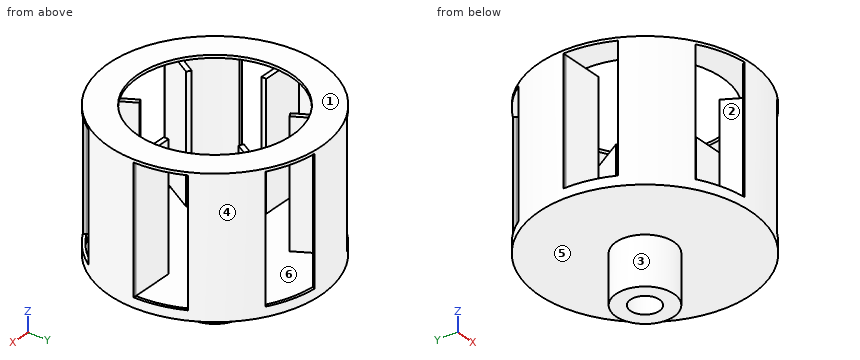
Autodesk Inventor part; units mm, degrees
ref_plane "Work Plane1" through (-58.9042, -102.025, 1.5) normal (-0.5, -0.866, 0) x (0.866, -0.5, 0)
ref_plane "YZ Plane" through (0, 0, 0) normal (1, 0, 0) x (0, 1, 0)
ref_plane "XZ Plane" through (0, 0, 0) normal (0, 1, 0) x (-1, 0, 0)
sketch "Sketch1" plane through (0, 0, 0) normal (0, 0, 1) x (1, 0, 0)
  circle A0 centre (0, 0) radius 55
  dimension "d0" = 110
extrude "Extrusion1" add sketch "Sketch1" along normal blind 71.5
shell "Shell1" thickness 1.5 removed faces 1 at (13.749, -10.4033, 71.5)
sketch "Sketch2" plane through (0, 0, 71.5) normal (0, 0, 1) x (1, 0, 0)
  circle A0 centre (0, 0) radius 55
  circle A1 centre (0, 0) radius 55
  circle A2 centre (0, 0) radius 40
  dimension "d4" = 110
  dimension "d5" = 80
extrude "Extrusion2" add sketch "Sketch2" against normal blind 1.5
sketch "Sketch3" plane through (0, 0, 0) normal (0, 0, -1) x (-1, 0, 0)
  circle A0 centre (0, 0) radius 15
  dimension "d8" = 30
extrude "Extrusion3" add sketch "Sketch3" along normal blind 25
sketch "Sketch4" plane through (0, 0, -25) normal (0, 0, -1) x (-1, 0, 0)
  circle A0 centre (0, 0) radius 7.5
  dimension "d11" = 15
extrude "Extrusion4" cut sketch "Sketch4" against normal blind 25
sketch "Sketch5" plane through (0, 0, 1.5) normal (0, 0, 1) x (1, 0, 0)
  circle A0 centre (0, 0) radius 7.5 construction
  line L0 (0, 0) -> (0, -95.8386) construction
  line L1 (0, 0) -> (-58.9042, -102.025)
  dimension "d14" = 30
ref_plane "Work Plane1" through (-58.9042, -102.025, 1.5) normal (-0.5, -0.866, 0) x (0.866, -0.5, 0)
sketch "Sketch7" plane through (-58.9042, -102.025, 1.5) normal (-0.5, -0.866, 0) x (0.866, -0.5, 0)
  line L0 (53.5, 0) -> (-53.5, 0)
  line L1 (55, -1.5) -> (-55, -1.5)
  line L2 (0, 3.5) -> (24, 3.5)
  line L3 (24, 3.5) -> (24, 68.5)
  line L4 (24, 68.5) -> (0, 68.5)
  line L5 (0, 68.5) -> (0, 3.5)
  line L6 (55, 70) -> (-55, 70)
  point P0 (0, -1.5)
  point P1 (0, -1.5)
  dimension "d18" = 5
  dimension "d19" = 65
  dimension "d20" = 24
  dimension "d21" = 0
  dimension "d22" = 1.5
extrude "Extrusion5" cut sketch "Sketch7" against normal blind 110.75
pattern_circular "Circular Pattern1" count 6 over 360 about axis through (0, 0, 0) along (0, 0, 1) of "Extrusion5"
sketch "Sketch12" plane through (0, 0, 5) normal (0, 0, 1) x (0.958, -0.2869, 0)
  line L0 (9.6549, 29.9119) -> (14.7648, 51.483)
  line L1 (14.7648, 51.483) -> (14.9013, 52.0593)
  line L2 (7.2222, 30.4881) -> (12.3321, 52.0593)
  line L3 (12.3321, 52.0593) -> (12.4686, 52.6356)
  line L4 (14.9013, 52.0593) -> (12.4686, 52.6356)
  line L5 (12.6779, 53.5189) -> (12.3321, 52.0593)
  line L6 (9.6549, 29.9119) -> (7.2222, 30.4881)
  point P0 (0, 0)
  point P1 (8.4385, 30.2)
  dimension "d34" = 2.5
  dimension "d35" = 30.2
extrude "Extrusion7" add sketch "Sketch12" along normal blind 65
pattern_circular "Circular Pattern2" count 6 over 360 about axis through (0, 0, -25) along (0, 0, 1) of "Extrusion7"
properties part number "Cilindro do Motor Industrial" material "Iron, Cast"
Verification items for the finished model (mm, model axes). Face numbers are marked on the shaded views. A direction names the side the tool comes from. Round coordinates to 2 decimals unless told otherwise and drop trailing zeros. Order: outer loops, then holes, each group sorted by start corner. A loop starts at its lowest first (then second) coordinate and runs counter-clockwise, first axis right, second up. Notation, with made-up numbers: (18, -28) - (50, -28) arc R13 cw to (50, -16) - close; hole circle Ø8 at (-27.75, 23.25). An arc over 180 degrees is marked (long way). Use CSV: the item, a comma, the result in double quotes. Start each with the question number.
1) Thickness scan on L1, parallel to Z at x = 21, y = -42.5; L2, parallel to Y at x = 0, z = 34.5; L3, parallel to Y at x = -19.5, z = 14. Record the ranges inside material, lowest first.
2) Section check C-C, the plane z = 58. State how many separate pieces and enclosed holes the cut face has, plus the area to 3 significant figures.
3) Section check D-D, the plane x = 0. Record the cut outline in (y, z), plus the area to 4 significant figures.
4) Section check B-B, the plane x = -35. Record the cut outline in (y, z), plus the area to 3 significant figures.
5) Access from +Z, -Z, +X, -X, +Y, -Y to the whole of each face (thin tool, end or side, straight path). Record for the marked faces 1, 2 and 3.
6) Go/stop test with flat-tipped pins: P1, Ø11, axis at x = 47, z = 31, coming from the +Y side; P2, Ø17.5, axis at x = -43, z = 34, coming from the -Y side; P3, Ø1, axis at y = -12, z = 20.5, coming from the +X side. Record where each tip stops, or that it passes through.
7) Section check A-A, the plane y = 9. Record the cut outline in (x, z), plus the area to 3 significant figures.
8) Mould release check, pull along X, two halves, no side actions. Record for the marked faces 4, 5 and 6: +X half, -X half, draft (parallel to the pull), parting line (faces both ways), or undercut.
Answers:
1,L1,"z = 0 to 1.5, 70 to 71.5"
1,L2,"y = -55 to -53.5, 53.5 to 55"
1,L3,"y = -33.78 to -28.78, 33.77 to 38.77, 49.82 to 51.43"
2,separate pieces,"6"
2,enclosed holes,"0"
2,area,"620 mm²"
3,outline,"(-55, 0) - (-15, 0) - (-15, -25) - (-7.5, -25) - (-7.5, 0) - (7.5, 0) - (7.5, -25) - (15, -25) - (15, 0) - (55, 0) - (55, 71.5) - (40, 71.5) - (40, 70) - (53.5, 70) - (53.5, 1.5) - (-53.5, 1.5) - (-53.5, 70) - (-40, 70) - (-40, 71.5) - (-55, 71.5) - close"
3,area,"790.5 mm²"
4,outline,"(-42.43, 0) - (42.43, 0) - (42.43, 5) - (40.46, 5) - (40.46, 1.5) - (-40.46, 1.5) - (-40.46, 70) - (-19.36, 70) - (-19.36, 71.5) - (-42.43, 71.5) - close; (0, 5) - (2.5, 5) - (2.5, 70) - (0, 70) - close; (19.36, 70) - (42.43, 70) - (42.43, 71.5) - (19.36, 71.5) - close"
4,area,"500 mm²"
5,face 1,"+Z, +X, -X, +Y, -Y"
5,face 2,"none"
5,face 3,"-Z"
6,P1,"stops at y = 36.09"
6,P2,"stops at y = -43.03"
6,P3,"stops at x = 53.78"
7,outline,"(-54.26, 0) - (-12, 0) - (-12, -25) - (12, -25) - (12, 0) - (54.26, 0) - (54.26, 5) - (52.74, 5) - (52.74, 1.5) - (-52.74, 1.5) - (-52.74, 70) - (-38.97, 70) - (-38.97, 71.5) - (-54.26, 71.5) - close; (38.97, 70) - (54.26, 70) - (54.26, 71.5) - (38.97, 71.5) - close"
7,area,"918 mm²"
8,face 4,"parting line"
8,face 5,"draft"
8,face 6,"undercut"
